```python
from build123d import *

# Parameters (mm, degrees)
SKETCH1_W           = 16
SKETCH1_H           = 21
SKETCH1_R           = 1.5
BOSS_EXTRUDE1_DEPTH = 1.6
SKETCH2_W           = 11
SKETCH2_H           = 10
BOSS_EXTRUDE2_DEPTH = 1.5
SKETCH3_W           = 12
SKETCH3_H           = 5
BOSS_EXTRUDE3_DEPTH = 2


with BuildPart() as part:
    # Sketch1 → Boss-Extrude1 (new body)
    with BuildSketch(Plane(origin=(0, 0, 0), x_dir=(1, 0, 0), z_dir=(0, 1, 0))):
        with Locations((8, 10.5)):
            Rectangle(SKETCH1_W, SKETCH1_H)
        with Locations(Location((3, 18, 0), (0, 0, 270))):
            Circle(SKETCH1_R, mode=Mode.SUBTRACT)
        with Locations(Location((13, 18, 0), (0, 0, 270))):
            Circle(SKETCH1_R, mode=Mode.SUBTRACT)
    extrude(amount=BOSS_EXTRUDE1_DEPTH)

    # Sketch2 → Boss-Extrude2 (add)
    with BuildSketch(Plane(origin=(0, 1.6, 0), x_dir=(1, 0, 0), z_dir=(0, 1, 0))):
        with Locations((9.5, 10)):
            Rectangle(SKETCH2_W, SKETCH2_H)
    extrude(amount=BOSS_EXTRUDE2_DEPTH)

    # Sketch3 → Boss-Extrude3 (add)
    with BuildSketch(Plane(origin=(0, 1.6, 0), x_dir=(1, 0, 0), z_dir=(0, 1, 0))):
        with Locations((8, 2.5)):
            Rectangle(SKETCH3_W, SKETCH3_H)
    extrude(amount=BOSS_EXTRUDE3_DEPTH)


solid = part.part
```
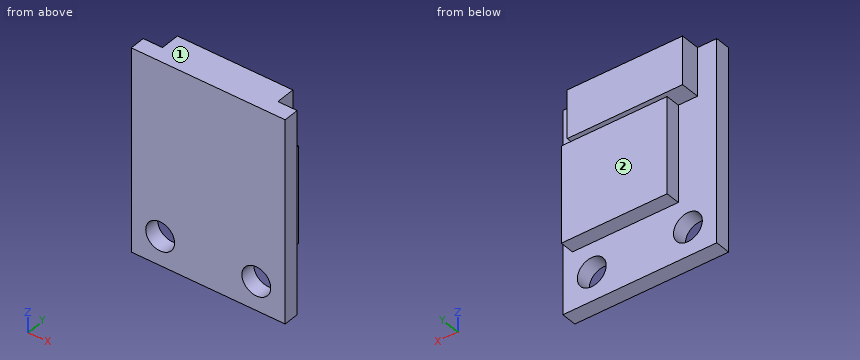
Input: part model. Units: mm. Frame: model coordinates. Face numbers are marked on the shaded views. A direction names the side the tool comes from. Coordinates: 2 decimals unless noted, no trailing zeros. Order: outer loops, then holes, each group sorted by start corner. A loop starts at its lowest first (then second) coordinate and runs counter-clockwise, first axis right, second up. Notation, with made-up numbers: (77.5, 84) - (87.5, 84) arc R20 cw to (87.5, 98) - close; hole circle Ø11 at (65.5, 72). An arc over 180 degrees is marked (long way). Put each result on its own line as item: value.
1. Line query: line 1 along X through (y, z) = (0.4, -18); line 2 along Y through (x, z) = (10.75, -12); line 3 along Z through (x, y) = (12.25, 2.3). Output: solid intervals per line, ascending.
Report:
line 1: x = 0 to 1.5, 4.5 to 11.5, 14.5 to 16
line 2: y = 0 to 3.1
line 3: z = -15 to 0
2. Cut plane C-C on y = 1.95. Return the cut outline in (x, z).
Report:
outline: (2, -5) - (4, -5) - (4, -15) - (15, -15) - (15, -5) - (14, -5) - (14, 0) - (2, 0) - close
3. Contact query for flat-ended pins moving along their axis: pin 1 Ø0.5 at (x, y) = (14.5, 2.5) entering from +Z; pin 2 Ø2 at (y, z) = (2.5, -2) entering from +X; pin 3 Ø8 at (x, z) = (10, -10.5) entering from +Y; pin 4 Ø0.8 at (x, y) = (7.5, 2.5) entering from -Z. Output: stop coordinate, or through.
Report:
pin 1: stops at z = -5
pin 2: stops at x = 16
pin 3: stops at y = 3.1
pin 4: stops at z = -15
4. Cut plane B-B on z = -18. Return the cut outline in (x, y).
Report:
outline: (0, 0) - (1.5, 0) - (1.5, 1.6) - (0, 1.6) - close; (4.5, 0) - (11.5, 0) - (11.5, 1.6) - (4.5, 1.6) - close; (14.5, 0) - (16, 0) - (16, 1.6) - (14.5, 1.6) - close
5. Cut plane A-A on x = 13. Return the cut outline in (y, z).
Report:
outline: (0, -21) - (1.6, -21) - (1.6, -19.5) - (0, -19.5) - close; (0, -16.5) - (1.6, -16.5) - (1.6, -15) - (3.1, -15) - (3.1, -5) - (3.6, -5) - (3.6, 0) - (0, 0) - close
6. Cut plane D-D on z = -1.25. Return the cut outline in (x, y), then the cut area to 3 significant figures.
Report:
outline: (0, 0) - (16, 0) - (16, 1.6) - (14, 1.6) - (14, 3.6) - (2, 3.6) - (2, 1.6) - (0, 1.6) - close
area: 49.6 mm2
7. Reachability of the marked faces 1 and 2 from +Z, -Z, +X, -X, +Y, -Y: full face, straight path, thin tool, end or side. Return the list, or none.
Report:
face 1: +Z, +X, -X, +Y, -Y
face 2: -Z, +X, -X, +Y
